from build123d import *

# Parameters (mm, degrees)
F1_DEPTH  = 31.75
F2_T      = -4
F3_W      = 4
F3_H      = 10
F4_DEPTH  = 63.5
F6_DEPTH  = 8
F8_DEPTH  = 2
F11_DEPTH = 4
F13_DEPTH = 4
F14_W     = 12.7
F14_H     = 4
F15_DEPTH = 10
F16_SIZE  = 5
F17_R     = 2.15
F18_DEPTH = 25
F19_W     = 30.1
F19_H     = 4


# Not quite as in the source:
# - a pattern or mirror of a feature is missing from the dataset's text; its kind, count and spacing are read off the source's solid


with BuildPart() as f1:
    # F0 (on Front) → F1 (new body, symmetric)
    with BuildSketch(Plane.XZ):
        Polygon((-10.35, 0), (10.35, 0), (10.35, 26.81), (6.35, 26.81), (-6.35, 26.81), (-10.35, 26.81), align=None)
    extrude(amount=F1_DEPTH, both=True)

    # F2
    f2_openings = [f1.faces().sort_by_distance(p)[0] for p in [
        (0, 0, 0),
    ]]
    offset(amount=F2_T, openings=f2_openings)

    # F3 (on face) → F4 (join, through all)
    with BuildSketch(Plane.XZ.offset(31.75)):
        with Locations((-8.35, 31.81)):
            Rectangle(F3_W, F3_H)
        with Locations((8.35, 31.81)):
            Rectangle(F3_W, F3_H)
    extrude(amount=-F4_DEPTH)

    # F5 (on Top) → F6 (join)
    with BuildSketch(Plane.XY):
        Polygon((-19.05, -23.05), (-10.35, -31.75), (-10.35, 31.75), (-19.05, 23.05), align=None)
        Polygon((10.35, 31.75), (10.35, -31.75), (19.05, -23.05), (19.05, 23.05), align=None)
    extrude(amount=F6_DEPTH)

    # F7 (on Front) → F8 (join, symmetric)
    with BuildSketch(Plane.XZ):
        Polygon((-19.05, 8), (-10.35, 8), (-10.35, 36.81), (-19.05, 28.11), align=None)
        Polygon((10.35, 8), (19.05, 8), (19.05, 28.11), (10.35, 36.81), align=None)
    f8 = extrude(amount=F8_DEPTH, both=True)

    # F8_copies: F8 across plane
    add(f8.mirror(Plane(origin=(0, -10.525, 0), x_dir=(0, 0, -1), z_dir=(0, -1, 0))))

    # F10 (on plane+point) → F11 (join)
    with BuildSketch(Plane.XZ.offset(-23.05)):
        Polygon((10.35, 8), (19.05, 8), (19.05, 28.11), (10.35, 36.81), align=None)
        Polygon((-19.05, 28.11), (-19.05, 8), (-10.35, 8), (-10.35, 36.81), align=None)
    extrude(amount=F11_DEPTH)

    # F12 (on face) → F13 (cut)
    with BuildSketch(Plane(origin=(0, 0, 0), x_dir=(1, 0, 0), z_dir=(0, 0, -1))):
        Polygon((-8.6931457505, -27.75), (8.6931457505, -27.75), (15.05, -21.3931457505), (15.05, 21.3931457505), (8.6931457505, 27.75), (-8.6931457505, 27.75), (-15.05, 21.3931457505), (-15.05, -21.3931457505), align=None)
    extrude(amount=-F13_DEPTH, mode=Mode.SUBTRACT)

    # F14 (on face) → F15 (join, through all)
    with BuildSketch(Plane.XY.offset(26.81)):
        with Locations((0, 29.75)):
            Rectangle(F14_W, F14_H)
    extrude(amount=F15_DEPTH)

    # F16
    f16_edges = [f1.edges().sort_by_distance(p)[0] for p in [
        (8.35, -31.75, 36.81),
        (-8.35, -31.75, 36.81),
    ]]
    chamfer(f16_edges, length=F16_SIZE)

    # F17 (on face) → F18 (cut)
    with BuildSketch(Plane.XY.offset(26.81)):
        with Locations((0, -10.525)):
            Circle(F17_R)
    extrude(amount=-F18_DEPTH, mode=Mode.SUBTRACT)

    # F19 (on face) → F20 (join, up to the next surface of F1)
    with BuildSketch(Plane(origin=(0, 0, 0), x_dir=(1, 0, 0), z_dir=(0, 0, -1))):
        with Locations((0, -10.525)):
            Rectangle(F19_W, F19_H)
    extrude(until=Until.NEXT, dir=(0, 0, 1))


solid = f1.part
The listing builds one solid part. Answer for the finished solid, in the listing's coordinates (mm). A direction names the side the tool comes from. Round coordinates to 2 decimals unless told otherwise and drop trailing zeros. Write each loop counter-clockwise with the first axis right and the second up, starting at its lowest first coordinate (ties: lowest second). Pieces come first, ordered by that corner, then holes. Notation, with made-up numbers: M 66,42.25 L 119,42.25 A18 cw 119,46.25 Z; hole C -23,12 d7. An arc over 180 degrees is marked long. Write each question's results on one line, items separated by ' | '. Start each with the question number.
(1) The part is cut by section B-B, the plane y = -6.5. Write down the section's boundary in (x, z).
(2) Find the intervals of material crossed by line 1 (Y direction, x = 3, z = 22.5) (3 decimals); line 2 (Y direction, x = 13, z = 13); line 3 (X direction, y = 19, z = 7), in increasing order.
(3) For faces 1 (the flat face through (0, -2, 26.81)), 2 (the flat face through (-15, 11, 8)), 3 (the flat face through (6.35, -10, 13)), determine the directions among +Z, -Z, +X, -X, +Y, -Y from which every point of the face is accessible in a straight line to the end or side of a thin tool.
(4) Each of these flat-tipped pins is pushed along its axis until it touches: P1, Ø4, axis at x = -7.5, y = -16, coming from the -Z side; P2, Ø4.5, axis at x = -14.5, z = 16, coming from the +Y side; P3, Ø3, axis at y = -4, z = 21, coming from the -X side. Where does it stop, or does it pass through?
(5) The part is cut by section A-A, the plane x = 0. Write down the section's boundary in (y, z) (3 decimals), and give its area (3 significant figures).
(6) Determine the mould class of faces 4 (the flat face through (19.05, 0, 11)), 5 (the flat face through (15.05, -6, 2)), 6 (the flat face through (-15, 19.05, 19)) for opening direction X: +X half, -X half, draft (parallel to the pull), parting line (faces both ways), or undercut.
Worked answers:
1) outline: M -19.05,0 L -15.05,0 L -15.05,4 L -6.35,4 L -6.35,22.81 L 6.35,22.81 L 6.35,4 L 15.05,4 L 15.05,0 L 19.05,0 L 19.05,8 L 10.35,8 L 10.35,36.81 L 6.35,36.81 L 6.35,26.81 L -6.35,26.81 L -6.35,36.81 L -10.35,36.81 L -10.35,8 L -19.05,8 Z
2) line 1: y = -31.75 to -27.75, 8.525 to 12.525, 27.75 to 31.75 | line 2: y = -23.05 to -19.05, -2 to 2, 19.05 to 23.05 | line 3: x = -19.05 to -6.35, 6.35 to 19.05
3) face 1: +Z, -Y | face 2: +Z, -X | face 3: -Z
4) P1: stops at z = 4 | P2: stops at y = 23.05 | P3: stops at x = -10.35
5) outline: M -31.75,0 L -27.75,0 L -27.75,22.81 L -12.675,22.81 L -12.675,26.81 L -31.75,26.81 Z; M -8.375,22.81 L 8.525,22.81 L 8.525,0 L 12.525,0 L 12.525,22.81 L 27.75,22.81 L 27.75,0 L 31.75,0 L 31.75,36.81 L 27.75,36.81 L 27.75,26.81 L -8.375,26.81 Z | area: 551 mm²
6) face 4: +X half | face 5: undercut | face 6: draft
